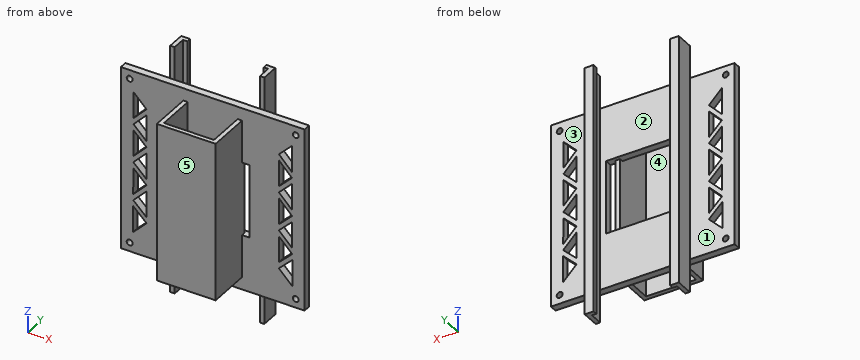
```python
from build123d import *

# Parameters (mm, degrees)
SKETCH_2_W               = 125
SKETCH_2_H               = 125
SKETCH_2_R               = 2
SKETCH_2_W_2             = 50
SKETCH_2_H_2             = 50
EXTRUDE_1_DEPTH          = 2.5
EXTRUDE_4_DEPTH          = 54
CUT_EXTRUDE_2_DEPTH      = 95.702164706
CUT_EXTRUDE_2_DEPTH_BACK = 5
EXTRUDE_7_DEPTH          = 85


with BuildPart() as part:
    # Sketch 2 → Extrude 1 (new, symmetric)
    with BuildSketch(Plane(origin=(0, 0, 0), x_dir=(1, 0, 0), z_dir=(0, 1, 0))):
        Rectangle(SKETCH_2_W, SKETCH_2_H)
        with Locations(Location((-56.5, 56.5, 0), (0, 0, 270))):
            Circle(SKETCH_2_R, mode=Mode.SUBTRACT)
        with Locations(Location((56.5, 56.5, 0), (0, 0, 270))):
            Circle(SKETCH_2_R, mode=Mode.SUBTRACT)
        with Locations(Location((-56.5, -56.5, 0), (0, 0, 270))):
            Circle(SKETCH_2_R, mode=Mode.SUBTRACT)
        with Locations(Location((56.5, -56.5, 0), (0, 0, 270))):
            Circle(SKETCH_2_R, mode=Mode.SUBTRACT)
        Rectangle(SKETCH_2_W_2, SKETCH_2_H_2, mode=Mode.SUBTRACT)
    extrude(amount=EXTRUDE_1_DEPTH, both=True)

    # Sketch 6 → Extrude 4 (add, symmetric)
    with BuildSketch(Plane.XY):
        Polygon((-20, 0), (-20, -31.5), (20, -31.5), (20, 0), (17, 0), (17, -28.5), (-17, -28.5), (-17, 0), align=None)
    extrude(amount=EXTRUDE_4_DEPTH, both=True)

    # Sketch 8 → Cut-Extrude 2 (cut, two sides: drawn at the far end of the back side and taken through both)
    with BuildSketch(Plane(origin=(0, 2.5, 0), x_dir=(1, 0, 0), z_dir=(0, 1, 0)).offset(-CUT_EXTRUDE_2_DEPTH_BACK)):
        Polygon((54.07931581, 22.285580831), (54.015526938, 4.28569386), (44.986382589, 13.073341514), align=None)
        Polygon((53.829622097, -48.172767848), (45.041121619, -39.384267369), (53.893419828, -30.170381277), align=None)
        Polygon((45.036831341, -35.272800588), (45.018048518, -17.272810388), (53.90806007, -26.039210725), align=None)
        Polygon((44.95901306, 39.30215881), (54.172270373, 48.515416123), (54.1084815, 30.515529152), align=None)
        Polygon((53.922585518, -21.940432956), (45.013752114, -13.155472476), (53.986361248, -3.944254461), align=None)
        Polygon((45.009460593, -9.042814869), (54.001004771, 0.18784173), (44.99067777, 8.957175331), align=None)
        Polygon((44.982089846, 17.187170851), (54.093962598, 26.418598199), (44.963307022, 35.187161051), align=None)
        Polygon((-53.893419828, -30.170381277), (-53.829622097, -48.172767848), (-45.041121619, -39.384267369), align=None)
        Polygon((-45.009460593, -9.042814869), (-44.99067777, 8.957175331), (-54.001004771, 0.18784173), align=None)
        Polygon((-53.986361248, -3.944254461), (-53.922585518, -21.940432956), (-45.013752114, -13.155472476), align=None)
        Polygon((-44.982089846, 17.187170851), (-44.963307022, 35.187161051), (-54.093962598, 26.418598199), align=None)
        Polygon((-54.1084815, 30.515529152), (-44.95901306, 39.30215881), (-54.172270373, 48.515416123), align=None)
        Polygon((-44.986382589, 13.073341514), (-54.07931581, 22.285580831), (-54.015526938, 4.28569386), align=None)
        Polygon((-53.90806007, -26.039210725), (-45.018048518, -17.272810388), (-45.036831341, -35.272800588), align=None)
    extrude(amount=CUT_EXTRUDE_2_DEPTH + CUT_EXTRUDE_2_DEPTH_BACK, mode=Mode.SUBTRACT)

    # Sketch 11 → Extrude 7 (add, symmetric)
    with BuildSketch(Plane.XY):
        Polygon((-32, 2.5), (-32, 14.5), (-26, 14.5), (-26, 11.5), (-29, 11.5), (-29, 2.5), align=None)
        Polygon((32, 2.5), (29, 2.5), (29, 11.5), (26, 11.5), (26, 14.5), (32, 14.5), align=None)
    extrude(amount=EXTRUDE_7_DEPTH, both=True)


solid = part.part
```
The listing builds one solid part. Answer for the finished solid, in the listing's coordinates (mm). Face numbers are marked on the shaded views. A direction names the side the tool comes from. Coordinates: 2 decimals unless noted, no trailing zeros. Write each loop counter-clockwise with the first axis right and the second up, starting at its lowest first coordinate (ties: lowest second). Pieces come first, ordered by that corner, then holes. Notation, with made-up numbers: (30, -4.5) - (71, -4.5) arc R31 ccw to (71, 24.5) - close; hole circle Ø9 at (-24, 73). An arc over 180 degrees is marked (long way). One line per item, written item: value.
1) Find section B-B (z = -56.5). Give the vertices of the cut face in (x, y), and give its area (3 significant figures).
Geometry check:
outline: (-62.5, -2.5) - (-58.5, -2.5) - (-58.5, 2.5) - (-62.5, 2.5) - close; (-54.5, -2.5) - (54.5, -2.5) - (54.5, 2.5) - (32, 2.5) - (32, 14.5) - (26, 14.5) - (26, 11.5) - (29, 11.5) - (29, 2.5) - (-29, 2.5) - (-29, 11.5) - (-26, 11.5) - (-26, 14.5) - (-32, 14.5) - (-32, 2.5) - (-54.5, 2.5) - close; (58.5, -2.5) - (62.5, -2.5) - (62.5, 2.5) - (58.5, 2.5) - close
area: 675 mm2
2) Each of these flat-tipped pins is pushed along its axis until it touches: pin 1 Ø4 at (y, z) = (-8, 44) entering from +X; pin 2 Ø2.5 at (y, z) = (6, 22) entering from +X; pin 3 Ø2.5 at (x, y) = (2, 0) entering from +Z; pin 4 Ø5 at (y, z) = (-23.5, 58.5) entering from -X. Where does it stop, or does it pass through?
Geometry check:
pin 1: stops at x = 20
pin 2: stops at x = 32
pin 3: stops at z = 62.5
pin 4: passes through
3) Find section A-A (x = 56.5). Give the vertices of the cut face in (y, z).
Geometry check:
outline: (-2.5, -62.5) - (2.5, -62.5) - (2.5, -58.5) - (-2.5, -58.5) - close; (-2.5, -54.5) - (2.5, -54.5) - (2.5, 54.5) - (-2.5, 54.5) - close; (-2.5, 58.5) - (2.5, 58.5) - (2.5, 62.5) - (-2.5, 62.5) - close
4) Consider line 1 along X through (y, z) = (-0.15, -56.5); line 2 along X through (y, z) = (0, -56); line 3 along X through (y, z) = (-25, 4). Determine where each line is inside the solid, lowest interval first. Write a range as from..to.
Geometry check:
line 1: x = -62.5..-58.5, -54.5..54.5, 58.5..62.5
line 2: x = -62.5..-58.44, -54.56..54.56, 58.44..62.5
line 3: x = -20..-17, 17..20
5) Find section D-D (z = 71.5). Give the vertices of the cut face in (x, y), and give its area (3 significant figures).
Geometry check:
outline: (-32, 2.5) - (-29, 2.5) - (-29, 11.5) - (-26, 11.5) - (-26, 14.5) - (-32, 14.5) - close; (26, 11.5) - (29, 11.5) - (29, 2.5) - (32, 2.5) - (32, 14.5) - (26, 14.5) - close
area: 90.0 mm2
6) A tool of negligible diameter and unlimited length cuts with its end or side. For the marked faces 1, 2 and 3, from which of +Z, -Z, +X, -X, +Y, -Y can it reach the whole face along a straight path? Write none if from no direction.
Geometry check:
face 1: +Z, -Z, -X, +Y
face 2: +Z, -Z
face 3: +Z, -Z, +X, +Y
7) Find section C-C (y = -20). Give the vertices of the cut face in (x, z).
Geometry check:
outline: (-20, -54) - (-17, -54) - (-17, 54) - (-20, 54) - close; (17, -54) - (20, -54) - (20, 54) - (17, 54) - close
8) For a pull along X with two mould halves and no side action, classify the marked faces 4 and 5 as pulls with the +X half, pulls with the -X half, needs draft (parallel to the pull), parting line crosses it, or undercut.
Geometry check:
face 4: undercut
face 5: needs draft
